Solid Edge part; units mm, degrees
sketch "Sketch1" plane through (0, 0, 0) normal (0, 0, 1) x (1, 0, 0)
  line L0 (27.5, 50) -> (27.5, -110)
  line L1 (27.5, -110) -> (-27.5, -110)
  line L2 (-27.5, -110) -> (-27.5, 50)
  line L3 (-27.5, 50) -> (27.5, 50)
  circle A0 centre (-15, 15) radius 1.25
  circle A1 centre (-15, -15) radius 1.25
  circle A2 centre (15, -15) radius 1.25
  circle A3 centre (15, 15) radius 1.25
extrude "Protrusion1" add sketch "Sketch1" along normal blind 5.5
fillet "Round_1" radius 10 4 edges at (27.5, 50, 2.75) (-27.5, 50, 2.75) (-27.5, -110, 2.75) (27.5, -110, 2.75)
sketch "Sketch2" plane through (0, 0, 0) normal (0, 0, 1) x (1, 0, 0)
  line L0 (23.5, -27.7908) -> (23.5, -37.7908)
  line L1 (23.5, -37.7908) -> (22.5, -37.7908)
  line L2 (22.5, -37.7908) -> (22.5, -27.7908)
  line L3 (22.5, -27.7908) -> (23.5, -27.7908)
  line L4 (23.5, -59.7908) -> (23.5, -69.7908)
  line L5 (23.5, -69.7908) -> (22.5, -69.7908)
  line L6 (22.5, -69.7908) -> (22.5, -59.7908)
  line L7 (22.5, -59.7908) -> (23.5, -59.7908)
  line L8 (23.5, -91.7908) -> (23.5, -101.7908)
  line L9 (23.5, -101.7908) -> (22.5, -101.7908)
  line L10 (22.5, -101.7908) -> (22.5, -91.7908)
  line L11 (22.5, -91.7908) -> (23.5, -91.7908)
extrude "Cutout1" cut sketch "Sketch2" along normal through all
mirror "Mirror1" about plane through (0, 0, 0) normal (1, 0, 0) of "Cutout1"
Here's how the part is built. I have some questions about the finished solid (model axes, mm). A direction names the side the tool comes from. Round coordinates to 2 decimals unless told otherwise and drop trailing zeros.
1. For faces 1 (the flat face through (-22.5, -65, 3)), 2 (the flat face through (0, -29, 0)), which set-ups out of +Z, -Z, +X, -X, +Y, -Y let a thin tool reach every point of the face, with its end or its side?
2. Will these pins go through, and if not, where does the flat tip stop? pin 1 Ø0.5 at (x, z) = (-23, 2.5) entering from +Y; pin 2 Ø0.8 at (x, z) = (23, 3.5) entering from -Y; pin 3 Ø0.8 at (x, z) = (-23, 1.5) entering from +Y.
3. If we mould it in two halves opening along Y, with no side actions, what happens to faces 3 (the cylindrical face through (24.49, -107.15, 2.79)), 4 (the cylindrical face through (-24.49, 47.15, 2.79)), 5 (the flat face through (-23.5, -33, 3)), 6 (the flat face through (0, -29, 5.5))? For each: released by +Y, released by -Y, zero draft, split by the parting line, or undercut.
4. Suppose I cut it at A-A (z = 3.7). State how many separate pieces and enclosed holes the cut face has, and give its area (3 significant figures).
5. I need wall thicknesses on L1, parallel to X at y = -92, z = 4.7; L2, parallel to Y at x = 15, z = 2.65; L3, parallel to X at y = -101, z = 5.1. Which ranges of each line are inside material? Lowest first, please.
Answer sheet:
1. face 1: +Z, -Z
1. face 2: -Z, +X, -X, +Y, -Y
2. pin 1: stops at y = 48.51
2. pin 2: stops at y = -108.6
2. pin 3: stops at y = 48.6
3. face 3: released by -Y
3. face 4: released by +Y
3. face 5: undercut
3. face 6: zero draft
4. separate pieces: 1
4. enclosed holes: 10
4. area: 8,630 mm2
5. L1: x = -27.5 to -23.5, -22.5 to 22.5, 23.5 to 27.5
5. L2: y = -110 to -16.25, -13.75 to 13.75, 16.25 to 50
5. L3: x = -27.45 to -23.5, -22.5 to 22.5, 23.5 to 27.45
